Source: three-view drawing plus pictorial views. Frame: mm from the lowest corner of the part. Give positions to 0.01 mm unless a question says otherwise; leave off trailing zeros. Loops run counter-clockwise (first coordinate to the right, second up) from the corner with the lowest first, then second, coordinate; pieces in that order, holes last. Notation, with made-up numbers: (9.25, 76) - (41.25, 76) arc R10 ccw to (41.25, 91) - close; hole circle Ø4 at (56, 86.25). An arc over 180 degrees is marked (long way). One line per item, written item: value.
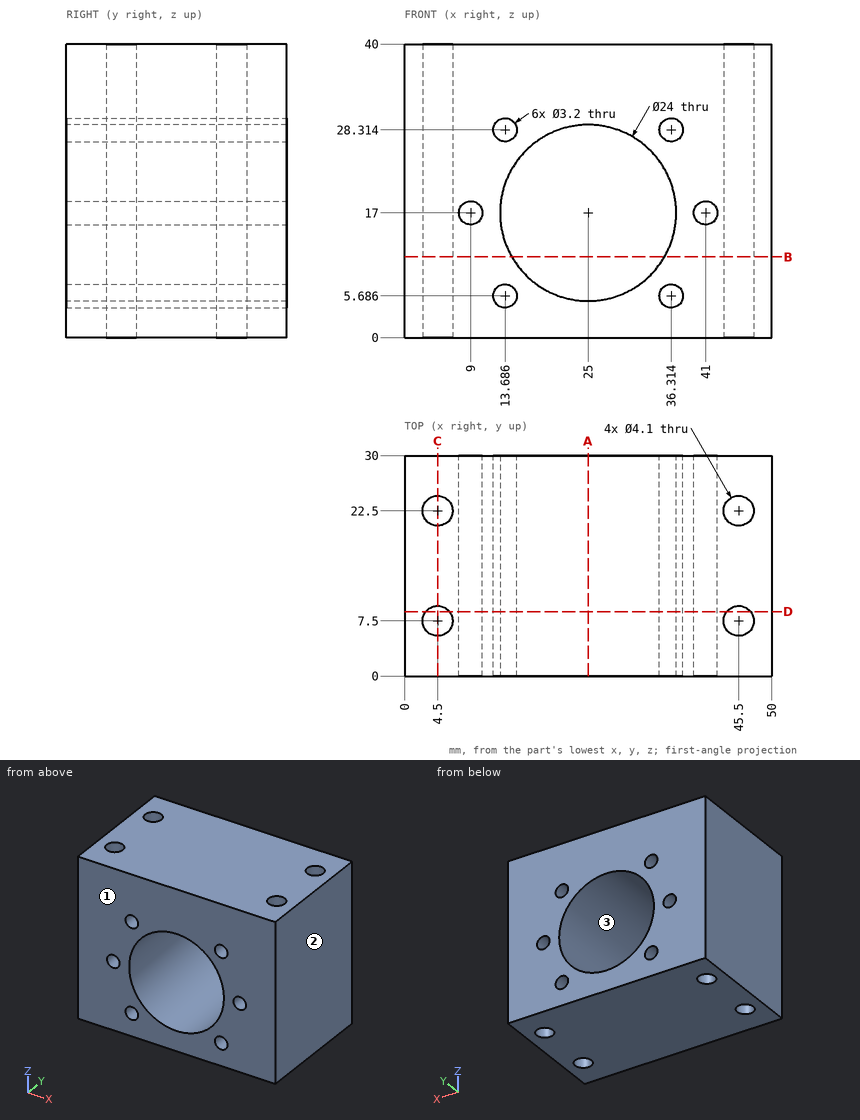
Item 1: Section D-D, the plane y = 8.75. Count the separate pieces of the cut face and the enclosed holes in it, and give its area (3 significant figures).
Verdict:
separate pieces: 3
enclosed holes: 7
area: 1,240 mm^2
Item 2: Draft query along X for the marked faces 1, 2 and 3. Return one class per face: pulls with the +X half, pulls with the -X half, needs draft (parallel to the pull), parting line crosses it, or undercut.
Verdict:
face 1: needs draft
face 2: pulls with the +X half
face 3: undercut
Item 3: Pin query (flat end, axial travel): P1, Ø3.5, axis at x = 45.5, y = 22.5, coming from the +Z side; P2, Ø5, axis at x = 36.31, z = 5.69, coming from the +Y side. Return the tip coordinate at first contact, or that it passes through.
Verdict:
P1: passes through
P2: stops at y = 30
Item 4: Section C-C, the plane x = 4.5. Output: boundary loops of the cut face in (y, z), and give its area (3 significant figures).
Verdict:
outline: (0, 0) - (5.45, 0) - (5.45, 40) - (0, 40) - close; (9.55, 0) - (20.45, 0) - (20.45, 40) - (9.55, 40) - close; (24.55, 0) - (30, 0) - (30, 40) - (24.55, 40) - close
area: 872 mm^2
Item 5: Material intervals for L1, parallel to X at y = 21, z = 16.5; L2, parallel to X at y = 15, z = 7 (1 decimal); L3, parallel to X at y = 20.75, z = 13 (1 decimal), sorted ascending.
Verdict:
L1: x = 0 to 3.1, 5.9 to 7.48, 10.52 to 13.01, 36.99 to 39.48, 42.52 to 44.1, 46.9 to 50
L2: x = 0 to 12.8, 14.6 to 18.4, 31.6 to 35.4, 37.2 to 50
L3: x = 0 to 3.4, 5.6 to 13.7, 36.3 to 44.4, 46.6 to 50
Item 6: Section B-B, the plane z = 11. Output: boundary loops of the cut face in (x, y).
Verdict:
outline: (0, 0) - (14.61, 0) - (14.61, 30) - (0, 30) - close; (35.39, 0) - (50, 0) - (50, 30) - (35.39, 30) - close; hole circle Ø4.1 at (4.5, 7.5); hole circle Ø4.1 at (4.5, 22.5); hole circle Ø4.1 at (45.5, 7.5); hole circle Ø4.1 at (45.5, 22.5)
Item 7: Section A-A, the plane x = 25. Output: boundary loops of the cut face in (y, z), and give its area (3 significant figures).
Verdict:
outline: (0, 0) - (30, 0) - (30, 5) - (0, 5) - close; (0, 29) - (30, 29) - (30, 40) - (0, 40) - close
area: 480 mm^2
